Geometry: final body of the model. Coordinates: model frame, mm. A direction names the side the tool comes from. Give positions to 0.01 mm unless a question says otherwise; leave off trailing zeros. Loops run counter-clockwise (first coordinate to the right, second up) from the corner with the lowest first, then second, coordinate; pieces in that order, holes last. Notation, with made-up numbers: M 74,69 L 97,69 A6 cw 97,75 Z; hole C 21,50.5 d3. An arc over 180 degrees is marked long. Put each result on its own line as item: value.
```python
from build123d import *

# Parameters (mm, degrees)
SKETCH_1_R          = 37.5
EXTRUDE_1_DEPTH     = 30
SKETCH_2_R          = 32.75
CUT_EXTRUDE_1_DEPTH = 14
CUT_EXTRUDE_2_DEPTH = 61.930288035


with BuildPart() as part:
    # 草图1 → 凸台-拉伸1 (new body)
    with BuildSketch(Plane(origin=(0, 0, 0), x_dir=(1, 0, 0), z_dir=(0, 1, 0))):
        with Locations(Location((0, 0, 0), (0, 0, 270))):
            Circle(SKETCH_1_R)
    extrude(amount=EXTRUDE_1_DEPTH)

    # 草图2 → 切除-拉伸1 (cut)
    with BuildSketch(Plane(origin=(0, 30, 0), x_dir=(1, 0, 0), z_dir=(0, 1, 0))):
        with Locations(Location((0, 0, 0), (0, 0, 270))):
            Circle(SKETCH_2_R)
    extrude(amount=-CUT_EXTRUDE_1_DEPTH, mode=Mode.SUBTRACT)

    # 草图3 → 切除-拉伸2 (cut, through all)
    with BuildSketch(Plane(origin=(0, 30, 0), x_dir=(1, 0, 0), z_dir=(0, 1, 0))):
        with BuildLine():
            Line((-35.443617197, 2), (-37.440440701, 2.112676056))
            ThreePointArc((-37.440440701, 2.112676056), (-37.485107218, 1.05675771), (-37.5, 0))
            Line((-37.5, 0), (-35.5, 0))
            ThreePointArc((-35.5, 0), (-35.4859015, 1.000397299), (-35.443617197, 2))
        make_face()
        with BuildLine():
            Line((-33.762506328, 10.9701033), (-35.664619361, 11.588137289))
            ThreePointArc((-35.664619361, 11.588137289), (-35.323899392, 12.588571472), (-34.955122297, 13.579006784))
            Line((-34.955122297, 13.579006784), (-33.090849107, 12.854793089))
            ThreePointArc((-33.090849107, 12.854793089), (-33.439958091, 11.917180994), (-33.762506328, 10.9701033))
        make_face()
        with BuildLine():
            Line((-28.7201033, 20.866376456), (-30.338137289, 22.041946961))
            ThreePointArc((-30.338137289, 22.041946961), (-29.704942178, 22.88812815), (-29.048152975, 23.716129717))
            Line((-29.048152975, 23.716129717), (-27.49891815, 22.451269465))
            ThreePointArc((-27.49891815, 22.451269465), (-28.120678595, 21.667427982), (-28.7201033, 20.866376456))
        make_face()
        with BuildLine():
            Line((-20.866376456, 28.7201033), (-22.041946961, 30.338137289))
            ThreePointArc((-22.041946961, 30.338137289), (-21.178258257, 30.947235372), (-20.29774805, 31.531752633))
            Line((-20.29774805, 31.531752633), (-19.215201487, 29.850059159))
            ThreePointArc((-19.215201487, 29.850059159), (-20.04875115, 29.296716153), (-20.866376456, 28.7201033))
        make_face()
        with BuildLine():
            Line((-10.9701033, 33.762506328), (-11.588137289, 35.664619361))
            ThreePointArc((-11.588137289, 35.664619361), (-10.57849886, 35.977011575), (-9.560458123, 36.260827907))
            Line((-9.560458123, 36.260827907), (-9.050567023, 34.326917085))
            ThreePointArc((-9.050567023, 34.326917085), (-10.014312254, 34.058237624), (-10.9701033, 33.762506328))
        make_face()
        with BuildLine():
            Line((0, 35.5), (0, 37.5))
            ThreePointArc((0, 37.5), (1.05675771, 37.485107218), (2.112676056, 37.440440701))
            Line((2.112676056, 37.440440701), (2, 35.443617197))
            ThreePointArc((2, 35.443617197), (1.000397299, 35.4859015), (0, 35.5))
        make_face()
        with BuildLine():
            Line((10.9701033, 33.762506328), (11.588137289, 35.664619361))
            ThreePointArc((11.588137289, 35.664619361), (12.588571472, 35.323899392), (13.579006784, 34.955122297))
            Line((13.579006784, 34.955122297), (12.854793089, 33.090849107))
            ThreePointArc((12.854793089, 33.090849107), (11.917180994, 33.439958091), (10.9701033, 33.762506328))
        make_face()
        with BuildLine():
            Line((20.866376456, 28.7201033), (22.041946961, 30.338137289))
            ThreePointArc((22.041946961, 30.338137289), (22.88812815, 29.704942178), (23.716129717, 29.048152975))
            Line((23.716129717, 29.048152975), (22.451269465, 27.49891815))
            ThreePointArc((22.451269465, 27.49891815), (21.667427982, 28.120678595), (20.866376456, 28.7201033))
        make_face()
        with BuildLine():
            Line((28.7201033, 20.866376456), (30.338137289, 22.041946961))
            ThreePointArc((30.338137289, 22.041946961), (30.947235372, 21.178258257), (31.531752633, 20.29774805))
            Line((31.531752633, 20.29774805), (29.850059159, 19.215201487))
            ThreePointArc((29.850059159, 19.215201487), (29.296716153, 20.04875115), (28.7201033, 20.866376456))
        make_face()
        with BuildLine():
            Line((33.762506328, 10.9701033), (35.664619361, 11.588137289))
            ThreePointArc((35.664619361, 11.588137289), (35.977011575, 10.57849886), (36.260827907, 9.560458123))
            Line((36.260827907, 9.560458123), (34.326917085, 9.050567023))
            ThreePointArc((34.326917085, 9.050567023), (34.058237624, 10.014312254), (33.762506328, 10.9701033))
        make_face()
        with BuildLine():
            Line((35.5, 0), (37.5, 0))
            ThreePointArc((37.5, 0), (37.485107218, -1.05675771), (37.440440701, -2.112676056))
            Line((37.440440701, -2.112676056), (35.443617197, -2))
            ThreePointArc((35.443617197, -2), (35.4859015, -1.000397299), (35.5, 0))
        make_face()
        with BuildLine():
            Line((33.762506328, -10.9701033), (35.664619361, -11.588137289))
            ThreePointArc((35.664619361, -11.588137289), (35.323899392, -12.588571472), (34.955122297, -13.579006784))
            Line((34.955122297, -13.579006784), (33.090849107, -12.854793089))
            ThreePointArc((33.090849107, -12.854793089), (33.439958091, -11.917180994), (33.762506328, -10.9701033))
        make_face()
        with BuildLine():
            Line((28.7201033, -20.866376456), (30.338137289, -22.041946961))
            ThreePointArc((30.338137289, -22.041946961), (29.704942178, -22.88812815), (29.048152975, -23.716129717))
            Line((29.048152975, -23.716129717), (27.49891815, -22.451269465))
            ThreePointArc((27.49891815, -22.451269465), (28.120678595, -21.667427982), (28.7201033, -20.866376456))
        make_face()
        with BuildLine():
            Line((20.866376456, -28.7201033), (22.041946961, -30.338137289))
            ThreePointArc((22.041946961, -30.338137289), (21.178258257, -30.947235372), (20.29774805, -31.531752633))
            Line((20.29774805, -31.531752633), (19.215201487, -29.850059159))
            ThreePointArc((19.215201487, -29.850059159), (20.04875115, -29.296716153), (20.866376456, -28.7201033))
        make_face()
        with BuildLine():
            Line((10.9701033, -33.762506328), (11.588137289, -35.664619361))
            ThreePointArc((11.588137289, -35.664619361), (10.57849886, -35.977011575), (9.560458123, -36.260827907))
            Line((9.560458123, -36.260827907), (9.050567023, -34.326917085))
            ThreePointArc((9.050567023, -34.326917085), (10.014312254, -34.058237624), (10.9701033, -33.762506328))
        make_face()
        with BuildLine():
            Line((0, -35.5), (0, -37.5))
            ThreePointArc((0, -37.5), (-1.05675771, -37.485107218), (-2.112676056, -37.440440701))
            Line((-2.112676056, -37.440440701), (-2, -35.443617197))
            ThreePointArc((-2, -35.443617197), (-1.000397299, -35.4859015), (0, -35.5))
        make_face()
        with BuildLine():
            Line((-10.9701033, -33.762506328), (-11.588137289, -35.664619361))
            ThreePointArc((-11.588137289, -35.664619361), (-12.588571472, -35.323899392), (-13.579006784, -34.955122297))
            Line((-13.579006784, -34.955122297), (-12.854793089, -33.090849107))
            ThreePointArc((-12.854793089, -33.090849107), (-11.917180994, -33.439958091), (-10.9701033, -33.762506328))
        make_face()
        with BuildLine():
            Line((-20.866376456, -28.7201033), (-22.041946961, -30.338137289))
            ThreePointArc((-22.041946961, -30.338137289), (-22.88812815, -29.704942178), (-23.716129717, -29.048152975))
            Line((-23.716129717, -29.048152975), (-22.451269465, -27.49891815))
            ThreePointArc((-22.451269465, -27.49891815), (-21.667427982, -28.120678595), (-20.866376456, -28.7201033))
        make_face()
        with BuildLine():
            Line((-28.7201033, -20.866376456), (-30.338137289, -22.041946961))
            ThreePointArc((-30.338137289, -22.041946961), (-30.947235372, -21.178258257), (-31.531752633, -20.29774805))
            Line((-31.531752633, -20.29774805), (-29.850059159, -19.215201487))
            ThreePointArc((-29.850059159, -19.215201487), (-29.296716153, -20.04875115), (-28.7201033, -20.866376456))
        make_face()
        with BuildLine():
            Line((-33.762506328, -10.9701033), (-35.664619361, -11.588137289))
            ThreePointArc((-35.664619361, -11.588137289), (-35.977011575, -10.57849886), (-36.260827907, -9.560458123))
            Line((-36.260827907, -9.560458123), (-34.326917085, -9.050567023))
            ThreePointArc((-34.326917085, -9.050567023), (-34.058237624, -10.014312254), (-33.762506328, -10.9701033))
        make_face()
    extrude(amount=-CUT_EXTRUDE_2_DEPTH, mode=Mode.SUBTRACT)


solid = part.part
```
Item 1: Pin query (flat end, axial travel): pin 1 Ø1 at (y, z) = (23.5, -28) entering from +X; pin 2 Ø3 at (x, y) = (9, 24.5) entering from +Z; pin 3 Ø3 at (y, z) = (26.5, -11.5) entering from +X. Return the tip coordinate at first contact, or that it passes through.
Output values:
pin 1: x = 25.5
pin 2: z = 36.74
pin 3: x = 35.66
Item 2: Line query: probe 1 along X at (y, z) = (16.5, -28.5); probe 2 along Z at (x, y) = (-9, 21); probe 3 along Y at (x, z) = (22, 16). Output: solid intervals per line, ascending. Write a range as [from, to].
Output values:
probe 1: [-24.37, -16.13], [16.13, 21.17], [23.27, 24.37]
probe 2: [-36.4, -31.49], [31.49, 36.4]
probe 3: [0, 16]
Item 3: Set-up query: faces 4 (the flat face through (-11.275, 15.21, 34.7)), 5 (the cylindrical face through (16.015, 14.79, 33.908)), 6 (the flat face through (36, 15, 0)), 7 (the flat face through (-2.057, 15.21, 36.456)), 8 (the cylindrical face through (-35.486, 15.21, -0.986)). Return all of +Z, -Z, +X, -X, +Y, -Y with unobstructed straight access to the full face (end or side cutting, diameter ignored); none if empty.
Output values:
face 4: +Y, -Y
face 5: +Z, +X, +Y, -Y
face 6: +X, +Y, -Y
face 7: +Z, +Y, -Y
face 8: -X, +Y, -Y
Item 4: Section A-A on x = 8. Output: boundary loops of the cut face in (y, z), then the cut area to 3 significant figures.
Output values:
outline: M 0,-36.64 L 30,-36.64 L 30,-31.76 L 16,-31.76 L 16,31.76 L 30,31.76 L 30,36.64 L 0,36.64 Z
area: 1,310 mm²
Item 5: Section B-B on z = 6. Output: boundary loops of the cut face in (x, y).
Output values:
outline: M -37.02,0 L 37.02,0 L 37.02,30 L 32.2,30 L 32.2,16 L -32.2,16 L -32.2,30 L -37.02,30 Z
Item 6: Mould query, pull axis X, two halves, no side actions, for faces 1 (the cylindrical face through (33.908, 14.79, -16.015)), 2 (the cylindrical face through (-25.71, 14.79, -27.3)), 3 (the flat face through (34.7, 15.21, 11.275)). Classes: pulls with the +X half, pulls with the -X half, needs draft (parallel to the pull), parting line crosses it, or undercut.
Output values:
face 1: pulls with the +X half
face 2: pulls with the -X half
face 3: undercut
